Build history of the part. All positions in model axes, mm. A direction names the side the tool comes from. Give positions to 0.01 mm unless a question says otherwise; leave off trailing zeros. Loops run counter-clockwise (first coordinate to the right, second up) from the corner with the lowest first, then second, coordinate; pieces in that order, holes last. Notation, with made-up numbers: (-6, 41) - (34, 41) arc R31 ccw to (34, 65) - close; hole circle Ø9 at (4, 10). An arc over 180 degrees is marked (long way). Return JSON: item names as keys, results as strings. Group by question number.
1) Slice it at A-A (x = 0). List the corners of the cut face in (y, z), and give its area (3 significant figures).
2) Mould opens along Z. For faces 1 (the face through (0, 0, 329.5)), 2 (the face through (-9, 0, 214.5)), 3 (the face through (-9, 0, 204.5)), 4 (the face through (0, 10, 284)) say: released by +Z, released by -Z, zero draft, split by the parting line, or undercut.
3) Slice it at C-C (z = 79). List the corners of the cut face in (x, y).
4) Drill centre lines: probe 1 along Z at (x, y) = (0, -9); probe 2 along Y at (x, z) = (-0.5, 17.5); probe 3 along X at (y, z) = (-1, 290.5). Where is each one in solid material? Low to high. Write a range as from..to.
5) 3-axis set-ups, long thin cutter, end or side, ignore diameter. For faces 5 (the face through (0, 10, 209)), 6 (the face through (4.57, 7.167, 246.545)), 7 (the face through (4.57, 7.167, 309.22)), 8 (the face through (10, 0, 284)), 9 (the face through (4.57, 7.167, 100.818)): which of +Z, -Z, +X, -X, +Y, -Y reach the whole face in a straight line?
6) Drop flat-ended pins along their axis: pin 1 (6 mm diameter, centred on x = 4, z = 194.5, fed in from +Y); pin 2 (6 mm diameter, centred on y = 2.5, z = 246.5, fed in from -X); pin 3 (10 mm diameter, centred on x = 1.5, z = 34.5, fed in from +Y); pin 4 (6 mm diameter, centred on x = 1.5, y = 1.5, fed in from -Z). Give the stop position or say it passes through.
```python
from build123d import *

# Parameters (mm, degrees)
SKETCH1_R           = 8.5
BOSS_EXTRUDE1_DEPTH = 329.5
SKETCH2_W           = 20
SKETCH2_H           = 20
BOSS_EXTRUDE2_DEPTH = 10
SKETCH3_W           = 20
SKETCH3_H           = 20
BOSS_EXTRUDE3_DEPTH = 10


with BuildPart() as part:
    # Sketch1 → Boss-Extrude1 (new body)
    with BuildSketch(Plane.XY):
        Circle(SKETCH1_R)
    extrude(amount=BOSS_EXTRUDE1_DEPTH)

    # Sketch2 → Boss-Extrude2 (add)
    with BuildSketch(Plane.XY.offset(279.5)):
        Rectangle(SKETCH2_W, SKETCH2_H)
    extrude(amount=BOSS_EXTRUDE2_DEPTH)

    # Sketch3 → Boss-Extrude3 (add)
    with BuildSketch(Plane.XY.offset(204.5)):
        Rectangle(SKETCH3_W, SKETCH3_H)
    extrude(amount=BOSS_EXTRUDE3_DEPTH)


solid = part.part
```
Results:
{
 "1": {"outline": "(-10, 204.5) - (-8.5, 204.5) - (-8.5, 0) - (8.5, 0) - (8.5, 204.5) - (10, 204.5) - (10, 214.5) - (8.5, 214.5) - (8.5, 279.5) - (10, 279.5) - (10, 289.5) - (8.5, 289.5) - (8.5, 329.5) - (-8.5, 329.5) - (-8.5, 289.5) - (-10, 289.5) - (-10, 279.5) - (-8.5, 279.5) - (-8.5, 214.5) - (-10, 214.5) - close", "area": "5,660 mm2"},
 "2": {"face 1": "released by +Z", "face 2": "undercut", "face 3": "released by -Z", "face 4": "zero draft"},
 "3": {"outline": "circle Ø17 at (0, 0)"},
 "4": {"probe 1": "204.5..214.5, 279.5..289.5", "probe 2": "-8.49..8.49", "probe 3": "-8.44..8.44"},
 "5": {"face 5": "+Z, -Z, +X, -X, +Y", "face 6": "none", "face 7": "+Z", "face 8": "+Z, -Z, +X, +Y, -Y", "face 9": "-Z"},
 "6": {"pin 1": "y = 8.44", "pin 2": "x = -8.5", "pin 3": "y = 8.5", "pin 4": "z = 0"}
}
